from build123d import *

# Parameters (mm, degrees)
SKETCH2_W           = 22.8
SKETCH2_H           = 7.5
BOSS_EXTRUDE1_DEPTH = 2.85
SKETCH3_R           = 3.35
BOSS_EXTRUDE2_DEPTH = 6.5
SKETCH4_RX          = 2.25
SKETCH4_RY          = 1.5
BOSS_EXTRUDE3_DEPTH = 9.8


with BuildPart() as part:
    # Sketch2 → Boss-Extrude1 (new body)
    with BuildSketch(Plane.XY):
        with Locations((11.4, 3.75)):
            Rectangle(SKETCH2_W, SKETCH2_H)
    extrude(amount=BOSS_EXTRUDE1_DEPTH)

    # Sketch3 → Boss-Extrude2 (add)
    with BuildSketch(Plane(origin=(22.8, 0, 0), x_dir=(0, 0, -1), z_dir=(1, 0, 0))):
        with Locations((-3.35, 3.75)):
            Circle(SKETCH3_R)
    extrude(amount=BOSS_EXTRUDE2_DEPTH)

    # Sketch4 → Boss-Extrude3 (add)
    with BuildSketch(Plane.ZY):
        with Locations(Location((1.5, 3.75), (0, 0, 90))):
            Ellipse(SKETCH4_RX, SKETCH4_RY)
    extrude(amount=BOSS_EXTRUDE3_DEPTH)


solid = part.part
Could you check a few things on this model? Use its own coordinates, in mm. A direction names the side the tool comes from. Round coordinates to 2 decimals unless told otherwise and drop trailing zeros. Order: outer loops, then holes, each group sorted by start corner. A loop starts at its lowest first (then second) coordinate and runs counter-clockwise, first axis right, second up. Notation, with made-up numbers: M 49,66.25 L 104,66.25 A23 cw 104,95.25 Z; hole C 39,36.5 d3. An arc over 180 degrees is marked long. One line per item, written item: value.
(1) If we mould it in two halves opening along X, with no side actions, what happens to faces 1 (the flat face through (0, 6.4, 1.4)), 2 (the flat face through (11, 4, 2.85)), 3 (the cylindrical face through (26.004, 6.014, 5.819)), 4 (the flat face through (22.8, 7, 1))? For each: released by +X, released by -X, zero draft, split by the parting line, or undercut.
Ans:
face 1: released by -X
face 2: undercut
face 3: zero draft
face 4: released by +X
(2) I'm going to push flat-ended pins straight in: P1, Ø1, axis at x = 22, z = 6, coming from the +Y side; P2, Ø1.2, axis at y = 5.5, z = 5, coming from the -X side; P3, Ø1.5, axis at x = 5.5, y = 1, coming from the -Z side. Where does each tip first touch, or does it pass through?
Ans:
P1: passes through
P2: stops at x = 22.8
P3: stops at z = 0
(3) Imagine slicing it at B-B (z = 3.35). Write out the boundary of the cut face in (x, y), and give its area (4 significant figures).
Ans:
outline: M 22.8,0.4 L 29.3,0.4 L 29.3,7.1 L 22.8,7.1 Z
area: 43.55 mm^2
(4) Which directions (+Z, -Z, +X, -X, +Y, -Y) give clear straight access to the entire face, cutting with the end or side of a thin tool? Please do faces 5 (the flat face through (11, 0, 1)), 6 (the flat face through (22.8, 1, 1)).
Ans:
face 5: +Z, -Z, +X, -X, -Y
face 6: -Z, +X, -Y
(5) I need wall thicknesses on line 1 along Z through (x, y) = (3, 5.5); line 2 along X through (y, z) = (3.25, 3); line 3 along X through (y, z) = (5.25, 2.75). Which ranges of each line are inside material? Lowest first, please. Write a range as from..to.
Ans:
line 1: z = 0..2.85
line 2: x = 22.8..29.3
line 3: x = 0..29.3
(6) Imagine slicing it at A-A (x = 18.5). Write out the boundary of the cut face in (y, z).
Ans:
outline: M 0,0 L 7.5,0 L 7.5,2.85 L 0,2.85 Z
